Build history of the part. All positions in model axes, mm. A direction names the side the tool comes from. Round coordinates to 2 decimals unless told otherwise and drop trailing zeros. Write each loop counter-clockwise with the first axis right and the second up, starting at its lowest first coordinate (ties: lowest second). Pieces come first, ordered by that corner, then holes. Notation, with made-up numbers: (-5.5, 51) -> (21.5, 51) arc R20 ccw to (21.5, 88) -> close; hole circle Ø8 at (76, 64). An arc over 180 degrees is marked (long way). Answer in a Markdown table with one row per item. Add a question column.
from build123d import *

# Parameters (mm, degrees)
SKETCH_1_R          = 3.5
EXTRUDE_1_DEPTH     = 5
FILLET_1_R          = 10
SKETCH_2_R          = 18
EXTRUDE_2_DEPTH     = 3
SKETCH_3_R          = 14
CUT_EXTRUDE_1_DEPTH = 32
SKETCH_4_R          = 16.75
CUT_EXTRUDE_2_DEPTH = 3
CHAMFER_1_SIZE      = 0.5


with BuildPart() as part:
    # 草图1 → 凸台-拉伸1 (new body)
    with BuildSketch(Plane.XY):
        with BuildLine():
            Line((-11.5, 18.165902125), (-7.564716302, 29.602895938))
            ThreePointArc((-7.564716302, 29.602895938), (0, 35), (7.564716302, 29.602895938))
            Line((7.564716302, 29.602895938), (11.5, 18.165902125))
            ThreePointArc((11.5, 18.165902125), (18.619546181, 10.75), (21.482132723, 0.876341081))
            Line((21.482132723, 0.876341081), (29.419218059, -8.250211479))
            ThreePointArc((29.419218059, -8.250211479), (30.310889132, -17.5), (21.854501757, -21.352684459))
            Line((21.854501757, -21.352684459), (9.982132723, -19.042243206))
            ThreePointArc((9.982132723, -19.042243206), (0, -21.5), (-9.982132723, -19.042243206))
            Line((-9.982132723, -19.042243206), (-21.854501757, -21.352684459))
            ThreePointArc((-21.854501757, -21.352684459), (-30.310889132, -17.5), (-29.419218059, -8.250211479))
            Line((-29.419218059, -8.250211479), (-21.482132723, 0.876341081))
            ThreePointArc((-21.482132723, 0.876341081), (-18.619546181, 10.75), (-11.5, 18.165902125))
        make_face()
        with Locations((0, 27)):
            Circle(SKETCH_1_R, mode=Mode.SUBTRACT)
        with Locations((23.382685902, -13.5)):
            Circle(SKETCH_1_R, mode=Mode.SUBTRACT)
        with Locations((-23.382685902, -13.5)):
            Circle(SKETCH_1_R, mode=Mode.SUBTRACT)
    extrude(amount=EXTRUDE_1_DEPTH)

    # 圆角1
    fillet_1_edges = [part.edges().sort_by_distance(p)[0] for p in [
        (21.482132723, 0.876341081, 2.5),
        (9.982132723, -19.042243206, 2.5),
        (-9.982132723, -19.042243206, 2.5),
        (-21.482132723, 0.876341081, 2.5),
        (-11.5, 18.165902125, 2.5),
        (11.5, 18.165902125, 2.5),
    ]]
    fillet(fillet_1_edges, radius=FILLET_1_R)

    # 草图2 → 凸台-拉伸2 (add)
    with BuildSketch(Plane.XY.offset(5)):
        Circle(SKETCH_2_R)
    extrude(amount=EXTRUDE_2_DEPTH)

    # 草图3 → 切除-拉伸1 (cut)
    with BuildSketch(Plane.XY.offset(8)):
        Circle(SKETCH_3_R)
    extrude(amount=-CUT_EXTRUDE_1_DEPTH, mode=Mode.SUBTRACT)

    # 草图4 → 切除-拉伸2 (cut)
    with BuildSketch(Plane(origin=(0, 0, 0), x_dir=(-1, 0, 0), z_dir=(0, 0, -1))):
        Circle(SKETCH_4_R)
    extrude(amount=-CUT_EXTRUDE_2_DEPTH, mode=Mode.SUBTRACT)

    # 倒角1
    chamfer_1_edges = [part.edges().sort_by_distance(p)[0] for p in [
        (-18, 0, 8),
    ]]
    chamfer(chamfer_1_edges, length=CHAMFER_1_SIZE)


solid = part.part
(1) Saw through at A-A (x = 0). List the corners of the cut face in (y, z), plus the area to 3 significant figures.
(2) Saw through at B-B (z = 4). List the corners of the cut face in (x, y), plus the area to 3 significant figures.
(3) Mould opens along Y. For faces 1 (the face through (26.616, -14.841, 2.465)), 2 (the face through (-18.67, 10.66, 2.46)), 3 (the face through (30.38, -17.38, 2.46)), 4 (the face through (4, -14, 3)) say: pulls with the +Y half, pulls with the -Y half, needs draft (parallel to the pull), parting line crosses it, or undercut.
(4) Saw through at C-C (y = 27). List the corners of the cut face in (x, z), plus the area to 3 significant figures.
(5) Saw through at D-D (x = -25.5). List the corners of the cut face in (y, z), plus the area to 3 significant figures.
(6) Drop flat-ended pins along their axis: P1, Ø12, axis at x = 9, y = 25.5, coming from the +Z side; P2, Ø4, axis at x = 20, z = 2, coming from the +Y side; P3, Ø1.5, axis at y = 21, z = 3.5, coming from the -X side. Give the stop position or say it passes through.
(7) Probe line 1 along Y through (x, z) = (0, 2.9); line 2 along Y through (x, z) = (0, 5.6); line 3 along Z through (x, y) = (-2, -18.5). List the from-to ranges inside material, lowest first.
(8) Which spindle directions (+Z, -Z, +X, -X, +Y, -Y) get a long thin tool onto all of the face, cutting with end or side? Do faces 5 (the face through (-26.523, -4.92, 2.465)), 6 (the face through (-17.399, -20.486, 2.465)), 7 (the face through (18.565, 10.844, 2.465)), 8 (the face through (3.63, -16.35, 1.48)), 9 (the face through (-2.343, 17.847, 6.232)). Say none if no direction does.
Answer sheet:
| question | item | result |
|---|---|---|
| 1 | outline | (-21.5, 0) -> (-16.75, 0) -> (-16.75, 3) -> (-14, 3) -> (-14, 8) -> (-17.5, 8) -> (-18, 7.5) -> (-18, 5) -> (-21.5, 5) -> close; (14, 3) -> (16.75, 3) -> (16.75, 0) -> (23.5, 0) -> (23.5, 5) -> (18, 5) -> (18, 7.5) -> (17.5, 8) -> (14, 8) -> close; (30.5, 0) -> (35, 0) -> (35, 5) -> (30.5, 5) -> close |
| 1 | area | 115 mm² |
| 2 | outline | (-29.42, -8.25) arc R8 ccw to (-21.85, -21.35) -> (-13.07, -19.64) arc R10 cw to (-7.61, -20.11) arc R21.5 ccw to (7.61, -20.11) arc R10 cw to (13.07, -19.64) -> (21.85, -21.35) arc R8 ccw to (29.42, -8.25) -> (23.54, -1.49) arc R10 cw to (21.22, 3.46) arc R21.5 ccw to (13.61, 16.65) arc R10 cw to (10.48, 21.14) -> (7.56, 29.6) arc R8 ccw to (-7.56, 29.6) -> (-10.48, 21.14) arc R10 cw to (-13.61, 16.65) arc R21.5 ccw to (-21.22, 3.46) arc R10 cw to (-23.54, -1.49) -> close; hole circle Ø7 at (-23.38, -13.5); hole circle Ø28 at (0, 0); hole circle Ø7 at (0, 27); hole circle Ø7 at (23.38, -13.5) |
| 2 | area | 1,400 mm² |
| 3 | face 1 | undercut |
| 3 | face 2 | pulls with the +Y half |
| 3 | face 3 | parting line crosses it |
| 3 | face 4 | undercut |
| 4 | outline | (-8.46, 0) -> (-3.5, 0) -> (-3.5, 5) -> (-8.46, 5) -> close; (3.5, 0) -> (8.46, 0) -> (8.46, 5) -> (3.5, 5) -> close |
| 4 | area | 49.6 mm² |
| 5 | outline | (-21.21, 0) -> (-16.29, 0) -> (-16.29, 5) -> (-21.21, 5) -> close; (-10.71, 0) -> (-3.74, 0) -> (-3.74, 5) -> (-10.71, 5) -> close |
| 5 | area | 59.5 mm² |
| 6 | P1 | stops at z = 5 |
| 6 | P2 | stops at y = 11.76 |
| 6 | P3 | stops at x = -10.83 |
| 7 | line 1 | y = -21.5 to -16.75, 16.75 to 23.5, 30.5 to 35 |
| 7 | line 2 | y = -18 to -14, 14 to 18 |
| 7 | line 3 | z = 0 to 5 |
| 8 | face 5 | +Z, -Z, -X, +Y |
| 8 | face 6 | +Z, -Z, -Y |
| 8 | face 7 | +Z, -Z, +X, +Y |
| 8 | face 8 | -Z |
| 8 | face 9 | +Z |
